The listing builds one solid part. Answer for the finished solid, in the listing's coordinates (mm). Face numbers are marked on the shaded views. Give positions to 0.01 mm unless a question says otherwise; leave off trailing zeros. Loops run counter-clockwise (first coordinate to the right, second up) from the corner with the lowest first, then second, coordinate; pieces in that order, holes last. Notation, with made-up numbers: (9, -13.5) - (46, -13.5) arc R22 ccw to (46, 19.5) - close; hole circle Ø4 at (77, 50.25). An arc over 180 degrees is marked (long way). Write item = value, one per line. Start each with the question number.
1) Consider probe 1 along X at (y, z) = (0, 15.5); probe 2 along Y at (x, z) = (-31.75, 17.75); probe 3 along Z at (x, y) = (-5.08, 0.25) (3 decimals). Determine where each line is inside the solid, lowest interval first.
2) The mould has two halves that part along Z. Classify the marked faces 1, 2, 3 and 4: +Z half, -Z half, draft (parallel to the pull), parting line (faces both ways), or undercut.
3) The part is cut by section C-C on y = 3. Write down the section's boundary in (x, z) (1 decimal).
4) The part is cut by section D-D on z = 15. Write down the section's boundary in (x, y), plus the area to 3 significant figures.
5) The part is cut by section A-A on x = -5.08. Write down the section's boundary in (y, z) (1 decimal), plus the area to 3 significant figures.
6) The part is cut by section B-B on z = 0. Write down the section's boundary in (x, y), plus the area to 3 significant figures.
from build123d import *

# Parameters (mm, degrees)
F0_W     = 76.2
F0_H     = 44.45
F1_DEPTH = 4.7625
F3_D     = 3.3
F3_DEPTH = 12
F3_TIP   = 0.9914200214
F5_D     = 6.6
F5_DEPTH = 12.7
F5_TIP   = 1.9828400428
F7_D     = 8.8


with BuildPart() as f1:
    # F0 (on Front) → F1 (new body, symmetric)
    with BuildSketch(Plane.XZ):
        Rectangle(F0_W, F0_H)
    extrude(amount=F1_DEPTH, both=True)

    # F3
    with Locations(Plane.XY.offset(22.225)):
        with Locations((-31.75, 0), (31.75, 0)):
            Hole(F3_D / 2, depth=F3_DEPTH)
            with Locations((0, 0, -(F3_DEPTH + F3_TIP / 2))):  # 118° drill point
                Cone(0, F3_D / 2, F3_TIP, mode=Mode.SUBTRACT)

    # F5
    with Locations(Plane.XZ.offset(4.7625)):
        with Locations((-28.8925, -1.905), (18.7325, -1.905)):
            Hole(F5_D / 2, depth=F5_DEPTH)
            with Locations((0, 0, -(F5_DEPTH + F5_TIP / 2))):  # 118° drill point
                Cone(0, F5_D / 2, F5_TIP, mode=Mode.SUBTRACT)

    # F7 (through all)
    with Locations(Plane.XZ.offset(4.7625)):
        with Locations((-5.08, -1.905)):
            Hole(F7_D / 2)


solid = f1.part
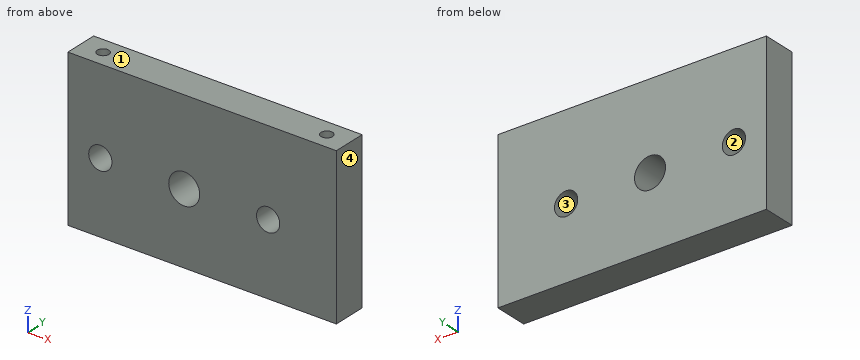
Answer below:
q1.probe_1 = -38.1 to -33.4, -30.1 to 30.1, 33.4 to 38.1
q1.probe_2 = -4.76 to -1.65, 1.65 to 4.76
q1.probe_3 = -22.225 to -6.305, 2.495 to 22.225
q2.face_1 = +Z half
q2.face_2 = undercut
q2.face_3 = undercut
q2.face_4 = draft
q3.outline = (-38.1, -22.2) - (38.1, -22.2) - (38.1, 22.2) - (-38.1, 22.2) - close; hole circle Ø6.6 at (-28.9, -1.9); hole circle Ø8.8 at (-5.1, -1.9); hole circle Ø6.6 at (18.7, -1.9)
q4.outline = (-38.1, -4.76) - (38.1, -4.76) - (38.1, 4.76) - (-38.1, 4.76) - close; hole circle Ø3.3 at (-31.75, 0); hole circle Ø3.3 at (31.75, 0)
q4.area = 709 mm2
q5.outline = (-4.8, -22.2) - (4.8, -22.2) - (4.8, -6.3) - (-4.8, -6.3) - close; (-4.8, 2.5) - (4.8, 2.5) - (4.8, 22.2) - (-4.8, 22.2) - close
q5.area = 340 mm2
q6.outline = (-38.1, -4.76) - (-31.59, -4.76) - (-31.59, 4.76) - (-38.1, 4.76) - close; (-26.2, -4.76) - (-9.05, -4.76) - (-9.05, 4.76) - (-26.2, 4.76) - close; (-1.11, -4.76) - (16.04, -4.76) - (16.04, 4.76) - (-1.11, 4.76) - close; (21.43, -4.76) - (38.1, -4.76) - (38.1, 4.76) - (21.43, 4.76) - close
q6.area = 548 mm2
